```python
from build123d import *

# Parameters (mm, degrees)
F1_DEPTH = 8.382
F3_DEPTH = 7.62


with BuildPart() as f1:
    # F0 (on Right) → F1 (new body)
    with BuildSketch(Plane.YZ):
        Polygon((133.310616, -138.339952), (-57.282638, 52.253302), (-57.282638, -138.339952), align=None)
    extrude(amount=F1_DEPTH)

    # F2 (on face) → F3 (join)
    with BuildSketch(Plane.YZ.offset(8.382)):
        Polygon((-57.282638, -133.343466), (-57.282638, -138.339952), (133.310616, -138.339952), (128.31413, -133.343466), align=None)
    extrude(amount=F3_DEPTH)


solid = f1.part
```
Design review of the part built by this model. Coordinates are the model's own, in mm. A direction names the side the tool comes from. Give positions to 0.01 mm unless a question says otherwise; leave off trailing zeros. Order: outer loops, then holes, each group sorted by start corner. A loop starts at its lowest first (then second) coordinate and runs counter-clockwise, first axis right, second up. Notation, with made-up numbers: (64, 29) -> (94, 29) arc R13 ccw to (94, 37) -> close; hole circle Ø4 at (-37.5, 82). An arc over 180 degrees is marked (long way). Write item = value, one per line. Start each with the question number.
(1) We need section B-B on x = 13. Write out the cut boundary in (y, z), plus the area to 3 significant figures.
(2) To check wall thickness, follow line 1 along X through (y, z) = (5, -17); line 2 along Z through (x, y) = (9.5, 57); line 3 along Z through (x, y) = (5, 108). State the ranges of each line that lie inside material, in increasing order.
(3) We need section A-A on y = 19.5. Write out the cut boundary in (x, z).
(4) For faces 1 (the face through (0, -6, -84)), 2 (the face through (8.382, -7, -80)), list the 3-axis set-ups (+Z, -Z, +X, -X, +Y, -Y) from which the entire face can be reached by the end or side of a thin tool; tool diameter is ignored.
(5) For pin 1 (4 mm diameter, centred on y = -34.5, z = -72, fed in from +X); pin 2 (6 mm diameter, centred on x = 10.5, z = -32, fed in from -Y); pin 3 (3 mm diameter, centred on x = 3, z = -104, fed in from +Y); pin 4 (1 mm diameter, centred on x = 2, y = 66.5, fed in from +Z), all flat-tipped, find the tip position at first contact; note any pin that passes through.
(6) We need section C-C on z = -119. Write out the cut boundary in (x, y), plus the area to 3 significant figures.
(7) We need section D-D on y = 53.5. Write out the cut boundary in (x, z).
Numbers:
q1.outline = (-57.28, -138.34) -> (133.31, -138.34) -> (128.31, -133.34) -> (-57.28, -133.34) -> close
q1.area = 940 mm^2
q2.line_1 = 0 to 8.38
q2.line_2 = -138.34 to -133.34
q2.line_3 = -138.34 to -113.03
q3.outline = (0, -138.34) -> (16, -138.34) -> (16, -133.34) -> (8.38, -133.34) -> (8.38, -24.53) -> (0, -24.53) -> close
q4.face_1 = +Z, -Z, -X, +Y, -Y
q4.face_2 = +Z, +X, +Y, -Y
q5.pin_1 = 8.38
q5.pin_2 = -57.28
q5.pin_3 = 100.47
q5.pin_4 = -71.03
q6.outline = (0, -57.28) -> (8.38, -57.28) -> (8.38, 113.97) -> (0, 113.97) -> close
q6.area = 1,440 mm^2
q7.outline = (0, -138.34) -> (16, -138.34) -> (16, -133.34) -> (8.38, -133.34) -> (8.38, -58.53) -> (0, -58.53) -> close
